from build123d import *

# Parameters (mm, degrees)
F0_W          = 101.6
F0_H          = 101.6
F1_DEPTH      = 1.27
F3_DEPTH      = 50.8
F3_DEPTH_BACK = 50.8
F4_W          = 12.7
F4_H          = 49.53
F5_DEPTH      = 1.27
F8_D          = 2.54
F9_R          = 2.54


with BuildPart() as f1:
    # F0 (on Top) → F1 (new body)
    with BuildSketch(Plane.XY):
        Rectangle(F0_W, F0_H)
    extrude(amount=F1_DEPTH)

    # F2 (on Right) → F3 (join, two sides)
    with BuildSketch(Plane.YZ) as f3_sk:
        Polygon((-68.1977470568, -18.5061718718), (-50.8, 0), (-51.7253085936, 0.8698873528), (-69.1230556503, -17.636284519), align=None)
        Polygon((-85.5954941135, -37.0123437436), (-68.1977470568, -18.5061718718), (-69.1230556503, -17.636284519), (-86.5208027071, -36.1424563908), align=None)
        Polygon((-51.7253085936, 0.8698873528), (-50.8, 0), (-50.8, 1.27), align=None)
    extrude(amount=F3_DEPTH)
    extrude(f3_sk.sketch, amount=-F3_DEPTH_BACK)

    # F4 (on face) → F5 (join)
    with BuildSketch(Plane(origin=(-50.8, 0, 0), x_dir=(0, -1, 0), z_dir=(-1, 0, 0))):
        with Locations((0, -24.765)):
            Rectangle(F4_W, F4_H)
    extrude(amount=-F5_DEPTH)

    # F6: F1 across plane


with BuildPart() as f1_1:
    add(f1.part)
    add(f1.part.mirror(Plane.YZ))

    # F8 (through all)
    with Locations(Plane(origin=(-50.8, 0, 0), x_dir=(0, -1, 0), z_dir=(-1, 0, 0))):
        with Locations((0, -40.7161329025)):
            Hole(F8_D / 2)

    # F9
    f9_edges = [f1_1.edges().sort_by_distance(p)[0] for p in [
        (0, -50.8, 0),
    ]]
    fillet(f9_edges, radius=F9_R)


solid = f1_1.part
Work out the finished part from the listing and answer in its coordinate system (mm). A direction names the side the tool comes from. Coordinates: 2 decimals unless noted, no trailing zeros. Loops run counter-clockwise (first coordinate to the right, second up) from the corner with the lowest first, then second, coordinate; pieces in that order, holes last. Notation, with made-up numbers: M 79,5.5 L 98,5.5 A18 ccw 98,17.5 Z; hole C 61.5,-23.5 d4. An arc over 180 degrees is marked long. Answer in a Markdown table with one row per item. Add a question column.
1. Flat-ended cylindrical pins translate along their axes: P1, Ø1.4, axis at x = 50, z = -20.5, coming from the -Y side; P2, Ø8, axis at x = 5, z = -9.5, coming from the +Y side; P3, Ø1.5, axis at x = -8.5, z = -7, coming from the +Y side; P4, Ø4, axis at y = 0, z = -40.72, coming from the -X side. Find the tip coordinate at first contact, or state that the pin passes through.
2. The mould has two halves that part along X. Classify faces 1 (the flat face through (-49.53, 0, -24)), 2 (the flat face through (-50.8, -3, -18)), 3 (the flat face through (-1, 1, 1.27)): pulls with the +X half, pulls with the -X half, needs draft (parallel to the pull), parting line crosses it, or undercut.
3. A tool of negligible diameter and unlimited length cuts with its end or side. For faces 4 (the flat face through (50.8, -3, -18)), 5 (the flat face through (49.53, 0, -24)), from which of +Z, -Z, +X, -X, +Y, -Y can it reach the whole face along a straight path? Write none if from no direction.
4. Find section A-A, the plane x = -30. Write down the section's boundary in (y, z), then the cut area to 3 significant figures.
5. Find section B-B, the plane y = -76.5. Write down the section's boundary in (x, z), then the cut area to 3 significant figures.
6. Find section C-C, the plane y = -14.5. Write down the section's boundary in (x, z), then the cut area to 3 significant figures.
7. Consider L1, parallel to Z at x = 50.4, y = 0; L2, parallel to Z at x = -31, y = -2; L3, parallel to Y at x = -25, z = -11.5. Determine where each line is inside the solid, lowest interval first.
Reported:
| question | item | result |
|---|---|---|
| 1 | P1 | stops at y = -72.47 |
| 1 | P2 | stops at y = -55.97 |
| 1 | P3 | stops at y = -56.68 |
| 1 | P4 | stops at x = -50.8 |
| 2 | face 1 | undercut |
| 2 | face 2 | pulls with the -X half |
| 2 | face 3 | needs draft |
| 3 | face 4 | +Z, -Z, +X, +Y, -Y |
| 3 | face 5 | -Z, +Y |
| 4 | outline | M -86.52,-36.14 L -85.6,-37.01 L -51.55,-0.8 A2.54 cw -49.7,0 L 50.8,0 L 50.8,1.27 L -50.8,1.27 L -51.73,0.87 Z |
| 4 | area | 194 mm^2 |
| 5 | outline | M -50.8,-27.34 L 50.8,-27.34 L 50.8,-25.48 L -50.8,-25.48 Z |
| 5 | area | 188 mm^2 |
| 6 | outline | M -50.8,0 L 50.8,0 L 50.8,1.27 L -50.8,1.27 Z |
| 6 | area | 129 mm^2 |
| 7 | L1 | z = -49.53 to -41.99, -39.45 to 1.27 |
| 7 | L2 | z = 0 to 1.27 |
| 7 | L3 | y = -63.35 to -61.61 |
